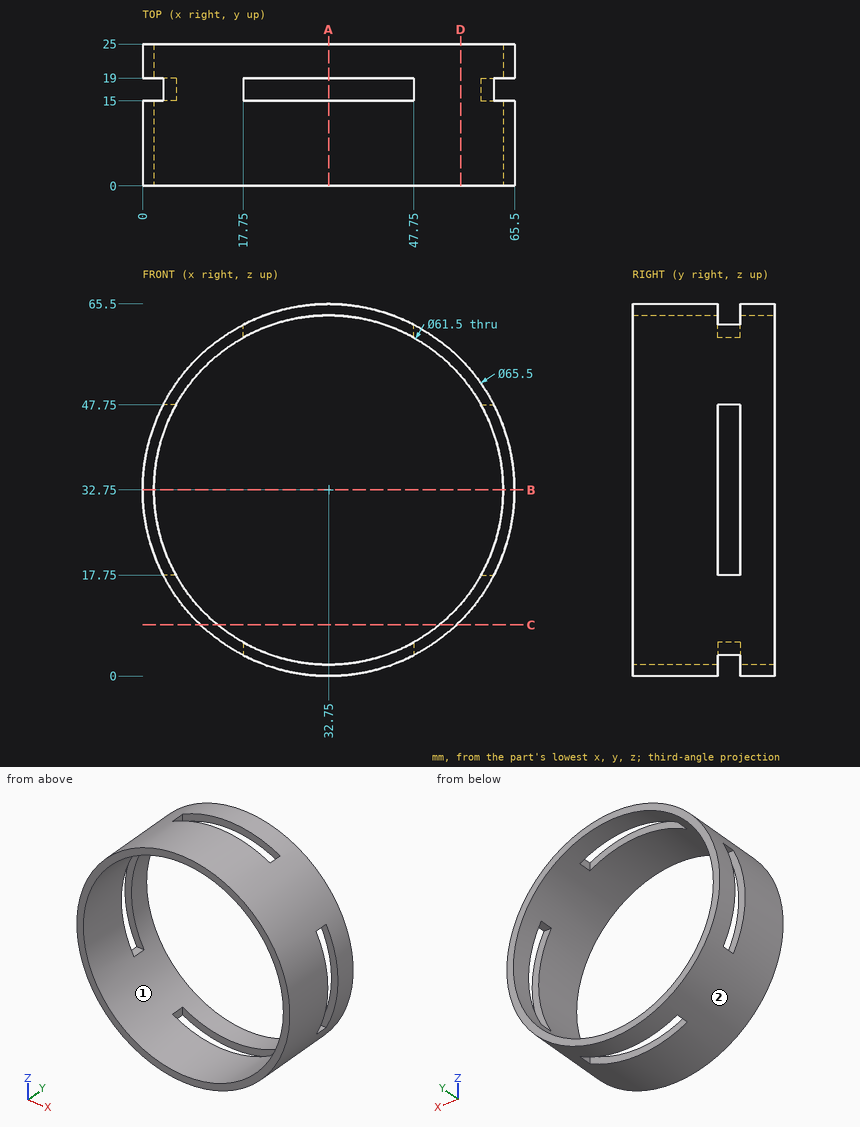
Drawing for the job (mm, zero at the part's lowest x, y, z). Coordinates: 2 decimals unless noted, no trailing zeros. Order: outer loops, then holes, each group sorted by start corner. A loop starts at its lowest first (then second) coordinate and runs counter-clockwise, first axis right, second up. Notation, with made-up numbers: (69, 30.5) - (80, 30.5) arc R11 cw to (80, 49.5) - close; hole circle Ø7 at (63, -6). An arc over 180 degrees is marked (long way). Use a Markdown table: item, result. Add a question column.
(1) Saw through at B-B (z = 32.75). Give the cut face in (x, y).
(2) Pull direction X, two halves, no side cores. Call the marked faces 1 and 2: +X half, -X half, draft (parallel to the pull), parting line (faces both ways), or undercut.
(3) Saw through at D-D (x = 56). Give the cut face in (y, z).
(4) Saw through at C-C (z = 9). Give the cut face in (x, y).
(5) Flat gauge pins, fed straight in: pin 1 (5 mm diameter, centred on y = 6, z = 20, fed in from -X); pin 2 (1 mm diameter, centred on x = 57.5, y = 22.5, fed in from -Z); pin 3 (10 mm diameter, centred on y = 13, z = 23.5, fed in from +X); pin 4 (1.8 mm diameter, centred on x = 62.5, z = 38, fed in from +Y). Where does each tip first touch, or does it go through?
(6) Drill centre lines: line 1 along Z through (x, y) = (32.75, 12.5); line 2 along X through (y, z) = (11.5, 22). Where is each one in solid material? Low to high. Write a range as [from, to].
(7) Saw through at A-A (x = 32.75). Give the cut face in (y, z).
Solved:
| question | item | result |
|---|---|---|
| 1 | outline | (0, 0) - (2, 0) - (2, 15) - (0, 15) - close; (0, 19) - (2, 19) - (2, 25) - (0, 25) - close; (63.5, 0) - (65.5, 0) - (65.5, 15) - (63.5, 15) - close; (63.5, 19) - (65.5, 19) - (65.5, 25) - (63.5, 25) - close |
| 2 | face 1 | undercut |
| 2 | face 2 | parting line |
| 3 | outline | (0, 9.68) - (25, 9.68) - (25, 12.63) - (0, 12.63) - close; (0, 52.87) - (25, 52.87) - (25, 55.82) - (0, 55.82) - close |
| 4 | outline | (10.2, 0) - (13.22, 0) - (13.22, 25) - (10.2, 25) - close; (52.28, 0) - (55.3, 0) - (55.3, 25) - (52.28, 25) - close |
| 5 | pin 1 | stops at x = 1.65 |
| 5 | pin 2 | stops at z = 10.74 |
| 5 | pin 3 | stops at x = 65.22 |
| 5 | pin 4 | stops at y = 25 |
| 6 | line 1 | z = [0, 2], [63.5, 65.5] |
| 6 | line 2 | x = [1.81, 3.94], [61.56, 63.69] |
| 7 | outline | (0, 0) - (15, 0) - (15, 2) - (0, 2) - close; (0, 63.5) - (15, 63.5) - (15, 65.5) - (0, 65.5) - close; (19, 0) - (25, 0) - (25, 2) - (19, 2) - close; (19, 63.5) - (25, 63.5) - (25, 65.5) - (19, 65.5) - close |
